Could you check a few things on this model? Use its own coordinates, in mm. Face numbers are marked on the shaded views. Round coordinates to 2 decimals unless told otherwise and drop trailing zeros. Write each loop counter-clockwise with the first axis right and the second up, starting at its lowest first coordinate (ties: lowest second). Pieces come first, ordered by that corner, then holes. Notation, with made-up numbers: (69.25, 26) -> (98.25, 26) arc R27 cw to (98.25, 60) -> close; hole circle Ø5 at (-25.5, 28). An arc over 180 degrees is marked (long way). Answer as CSV lines item,"result". Start each with the question number.
Q1. Will these pins go through, and if not, where does the flat tip stop? pin 1 Ø1.2 at (y, z) = (-11, 2) entering from -X; pin 2 Ø1.8 at (x, y) = (-27.5, -6) entering from +Z; pin 3 Ø2 at (x, y) = (-33.17, -1) entering from -Z; pin 4 Ø1.2 at (y, z) = (-12.5, 1.5) entering from +X.
Q2. Imagine slicing it at A-A on x = 12.5. Please give me the cut outline in (y, z).
Q3. If we mould it in two halves opening along Y, with no side actions, what happens to the marked faces 1, 2 and 3? For each: pulls with the +Y half, pulls with the -Y half, needs draft (parallel to the pull), parting line crosses it, or undercut.
Q4. If I drill on line 1 (X direction, y = -14.75, z = -1.5); line 2 (Z direction, x = -58, y = -12.3); line 3 (Y direction, x = -25.4, z = -4.05), over which ranges is the centre line in solid material (lowest first)? Write a range as [from, to].
from build123d import *

# Parameters (mm, degrees)
SKETCH_W            = 124
SKETCH_H            = 18.5
SKETCH_R            = 0.5
PAD_DEPTH           = 6
HOLE_D              = 0.7
HOLE_DEPTH          = 25
HOLE_CBORE_D        = 1.6
HOLE_CBORE_DEPTH    = 2.1
CHAMFER_SIZE        = 0.2
SKETCH002_W         = 12
SKETCH002_H         = 18.5
SKETCH002_W_2       = 36
SKETCH002_H_2       = 3
PAD001_DEPTH        = 4
CHAMFER001_SIZE     = 0.4
SKETCH003_R         = 1.1
POCKET_DEPTH        = 10.001
CHAMFER002_SIZE     = 0.7
SKETCH004_W         = 8
SKETCH004_H         = 8.5
POCKET001_DEPTH     = 8
HOLE003_D           = 2
HOLE003_CBORE_D     = 4.1
HOLE003_CBORE_DEPTH = 2.1
FILLET_R            = 4
POCKET002_DEPTH     = 2.1
SKETCH022_W         = 11.69728
SKETCH022_H         = 8
POCKET005_DEPTH     = 3
SKETCH023_W         = 11.69728
SKETCH023_H         = 5
POCKET006_DEPTH     = 5


with BuildPart() as part:
    # Sketch → Pad (new body)
    with BuildSketch(Plane(origin=(0, 0, 0), x_dir=(-1, 0, 0), z_dir=(0, 0, -1))):
        with Locations((0, -6.75)):
            Rectangle(SKETCH_W, SKETCH_H)
        with Locations((-33.67, -3.81)):
            Circle(SKETCH_R, mode=Mode.SUBTRACT)
        with Locations((-31.745, -3.81)):
            Circle(SKETCH_R, mode=Mode.SUBTRACT)
        with Locations((-21.595, -3.81)):
            Circle(SKETCH_R, mode=Mode.SUBTRACT)
        with Locations((-19.67, -3.81)):
            Circle(SKETCH_R, mode=Mode.SUBTRACT)
        with Locations((19.67, -3.81)):
            Circle(SKETCH_R, mode=Mode.SUBTRACT)
        with Locations((21.595, -3.81)):
            Circle(SKETCH_R, mode=Mode.SUBTRACT)
        with Locations((31.745, -3.81)):
            Circle(SKETCH_R, mode=Mode.SUBTRACT)
        with Locations((33.67, -3.81)):
            Circle(SKETCH_R, mode=Mode.SUBTRACT)
    extrude(amount=PAD_DEPTH)

    # Hole
    with Locations(Plane.XY):
        with Locations((-30.48, -6.25), (-27.94, -6.25), (-25.4, -6.25), (-22.86, -6.25), (22.86, -6.25), (25.4, -6.25), (27.94, -6.25), (30.48, -6.25)):
            CounterBoreHole(HOLE_D / 2, HOLE_CBORE_D / 2, HOLE_CBORE_DEPTH, depth=HOLE_DEPTH)

    # Chamfer
    chamfer_edges = [part.edges().sort_by_distance(p)[0] for p in [
        (30.13, -6.25, -2.1),
        (27.59, -6.25, -2.1),
        (25.05, -6.25, -2.1),
        (22.51, -6.25, -2.1),
        (-30.83, -6.25, -2.1),
        (-28.29, -6.25, -2.1),
        (-25.75, -6.25, -2.1),
        (-23.21, -6.25, -2.1),
    ]]
    chamfer(chamfer_edges, length=CHAMFER_SIZE)

    # Sketch002 (on Face25 of Chamfer) → Pad001 (join)
    with BuildSketch(Plane.XY):
        with Locations((-56, -6.75)):
            Rectangle(SKETCH002_W, SKETCH002_H)
        with Locations((56, -6.75)):
            Rectangle(SKETCH002_W, SKETCH002_H)
        with Locations((0, 1)):
            Rectangle(SKETCH002_W_2, SKETCH002_H_2)
        Polygon((-46, -16), (-46, -8), (-43, -8), (-43, -13), (-36, -13), (-36, -16), align=None)
        Polygon((46, -16), (46, -8), (43, -8), (43, -13), (36, -13), (36, -16), align=None)
    extrude(amount=PAD001_DEPTH)

    # Chamfer001
    chamfer001_edges = [part.edges().sort_by_distance(p)[0] for p in [
        (34.17, -3.81, -6),
        (32.245, -3.81, -6),
        (22.095, -3.81, -6),
        (20.17, -3.81, -6),
        (-19.17, -3.81, -6),
        (-21.095, -3.81, -6),
        (-31.245, -3.81, -6),
        (-33.17, -3.81, -6),
    ]]
    chamfer(chamfer001_edges, length=CHAMFER001_SIZE)

    # Sketch003 (on Face23 of Chamfer001) → Pocket (cut, through all)
    with BuildSketch(Plane.XY.offset(4)):
        with Locations((-33.17, -1)):
            Circle(SKETCH003_R)
        with Locations((-20.17, -1)):
            Circle(SKETCH003_R)
        with Locations((-33.17, -6.75)):
            Circle(SKETCH003_R)
        with Locations((-20.17, -6.75)):
            Circle(SKETCH003_R)
        with Locations((-20.17, -12.5)):
            Circle(SKETCH003_R)
        with Locations((-33.17, -12.5)):
            Circle(SKETCH003_R)
        with Locations((20.17, -1)):
            Circle(SKETCH003_R)
        with Locations((33.17, -1)):
            Circle(SKETCH003_R)
        with Locations((20.17, -6.75)):
            Circle(SKETCH003_R)
        with Locations((33.17, -6.75)):
            Circle(SKETCH003_R)
        with Locations((33.17, -12.5)):
            Circle(SKETCH003_R)
        with Locations((20.17, -12.5)):
            Circle(SKETCH003_R)
    extrude(amount=-POCKET_DEPTH, mode=Mode.SUBTRACT)

    # Chamfer002
    chamfer002_edges = [part.edges().sort_by_distance(p)[0] for p in [
        (19.07, -6.75, -6),
        (19.07, -1, -6),
        (19.07, -12.5, -6),
        (32.07, -12.5, -6),
        (32.07, -6.75, -6),
        (32.07, -1, -6),
        (-34.27, -1, -6),
        (-34.27, -6.75, -6),
        (-34.27, -12.5, -6),
        (-21.27, -12.5, -6),
        (-21.27, -6.75, -6),
        (-21.27, -1, -6),
    ]]
    chamfer(chamfer002_edges, length=CHAMFER002_SIZE)

    # Sketch004 (on Face35 of Chamfer002) → Pocket001 (cut)
    with BuildSketch(Plane.XY.offset(4)):
        with Locations((-58, -6.75)):
            Rectangle(SKETCH004_W, SKETCH004_H)
        with Locations((58, -6.75)):
            Rectangle(SKETCH004_W, SKETCH004_H)
    extrude(amount=-POCKET001_DEPTH, mode=Mode.SUBTRACT)

    # Hole003 (through all)
    with Locations(Plane.XZ.offset(16)):
        with Locations((-58, 0), (58, 0)):
            CounterBoreHole(HOLE003_D / 2, HOLE003_CBORE_D / 2, HOLE003_CBORE_DEPTH)

    # Fillet
    fillet_edges = [part.edges().sort_by_distance(p)[0] for p in [
        (-62, 0, 4),
        (-62, -13.5, 4),
        (62, 0, 4),
        (62, -13.5, 4),
        (54, -6.75, -4),
        (-54, -6.75, -4),
    ]]
    fillet(fillet_edges, radius=FILLET_R)

    # Sketch015 (on Face1 of Fillet) → Pocket002 (cut)
    with BuildSketch(Plane(origin=(0, 2.5, 0), x_dir=(-1, 0, 0), z_dir=(0, 1, 0))):
        Polygon((-56.845299, 2), (-59.154701, 2), (-60.309401, 0), (-59.154701, -2), (-56.845299, -2), (-55.690599, 0), align=None)
        Polygon((55.690599, 0), (56.845299, -2), (59.154701, -2), (60.309401, 0), (59.154701, 2), (56.845299, 2), align=None)
    extrude(amount=-POCKET002_DEPTH, mode=Mode.SUBTRACT)

    # Sketch022 (on Face4 of Pocket002) → Pocket005 (cut)
    with BuildSketch(Plane(origin=(0, 0, -6), x_dir=(1, 0, 0), z_dir=(0, 0, -1))):
        with Locations((0, 8)):
            Rectangle(SKETCH022_W, SKETCH022_H)
    extrude(amount=-POCKET005_DEPTH, mode=Mode.SUBTRACT)

    # Sketch023 (on Face122 of Pocket005) → Pocket006 (cut)
    with BuildSketch(Plane(origin=(0, 0, -3), x_dir=(1, 0, 0), z_dir=(0, 0, -1))):
        with Locations((0, 6.5)):
            Rectangle(SKETCH023_W, SKETCH023_H)
    extrude(amount=-POCKET006_DEPTH, mode=Mode.SUBTRACT)


solid = part.part
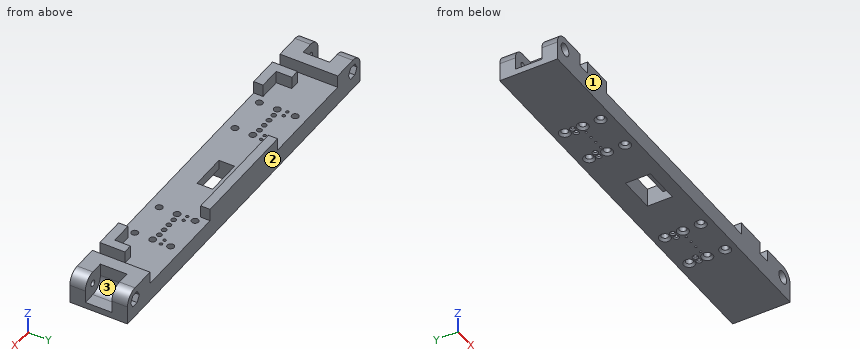
Checks:
1,pin 1,"x = -61.75"
1,pin 2,"z = 0"
1,pin 3,"through"
1,pin 4,"x = 61.9"
2,outline,"(-16, -6) -> (2.5, -6) -> (2.5, 4) -> (-0.5, 4) -> (-0.5, 0) -> (-16, 0) -> close"
3,face 1,"pulls with the -Y half"
3,face 2,"pulls with the +Y half"
3,face 3,"undercut"
4,line 1,"[-62, -59.4], [-56.6, 56.6], [59.4, 62]"
4,line 2,"[-6, -1], [1, 4]"
4,line 3,"[-16, -6.6], [-5.9, 2.5]"
